Verification items for the finished model (mm, model axes). Face numbers are marked on the shaded views. A direction names the side the tool comes from. Round coordinates to 2 decimals unless told otherwise and drop trailing zeros. Write each loop counter-clockwise with the first axis right and the second up, starting at its lowest first coordinate (ties: lowest second). Pieces come first, ordered by that corner, then holes. Notation, with made-up numbers: (-29.75, -13) - (1.25, -13) arc R27 ccw to (1.25, 13) - close; hole circle Ø9 at (40.25, 28.25). An arc over 180 degrees is marked (long way). Write each question's results on one line, items separated by ' | '.
```python
from build123d import *

# Parameters (mm, degrees)
F1_DEPTH = 4
F3_DEPTH = 2
F4_R     = 1


with BuildPart() as f1:
    # F0 (on Top) → F1 (new body)
    with BuildSketch(Plane.XY):
        with BuildLine():
            ThreePointArc((-5, 0), (0, -5), (5, 0))
            ThreePointArc((5, 0), (0, 5), (-5, 0))
        make_face()
        Polygon((-4.041452, 0), (-2.020726, 3.5), (2.020726, 3.5), (4.041452, 0), (2.020726, -3.5), (-2.020726, -3.5), align=None, mode=Mode.SUBTRACT)
        with BuildLine():
            Line((5, -45), (5, 0))
            ThreePointArc((5, 0), (0, -5), (-5, 0))
            Line((-5, 0), (-5, -45))
            ThreePointArc((-5, -45), (0, -50), (5, -45))
        make_face()
    extrude(amount=F1_DEPTH)

    # F2 (on face) → F3 (cut)
    with BuildSketch(Plane.XY.offset(4)):
        with BuildLine():
            ThreePointArc((2.5, -9), (0, -6.5), (-2.5, -9))
            Line((-2.5, -9), (-2.5, -45))
            ThreePointArc((-2.5, -45), (0, -47.5), (2.5, -45))
            Line((2.5, -45), (2.5, -9))
        make_face()
    extrude(amount=-F3_DEPTH, mode=Mode.SUBTRACT)

    # F4
    f4_edges = [f1.edges().sort_by_distance(p)[0] for p in [
        (0, -6.5, 2),
        (-2.5, -27, 2),
        (0, -47.5, 2),
        (2.5, -27, 2),
    ]]
    fillet(f4_edges, radius=F4_R)


solid = f1.part
```
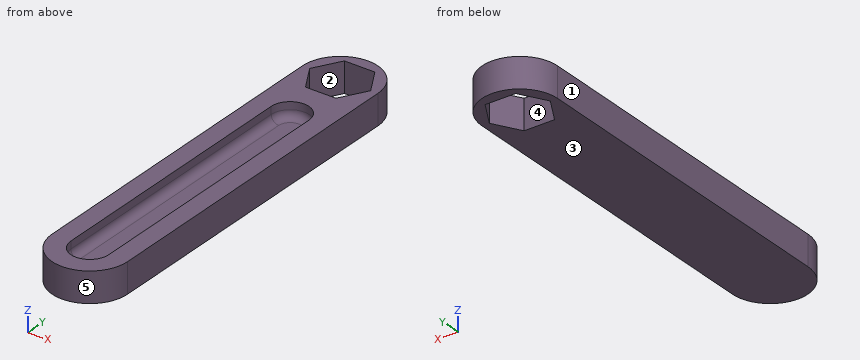
(1) Section check B-B (z = 1.3). Record the cut outline in (x, y), plus the area to 3 significant figures.
Answer:
outline: (-5, -45) arc R5 ccw to (5, -45) - (5, 0) arc R5 ccw to (-5, 0) - close; hole (-4.04, 0) - (-2.02, -3.5) - (2.02, -3.5) - (4.04, 0) - (2.02, 3.5) - (-2.02, 3.5) - close | area: 486 mm2
(2) Section check A-A (x = 0). Record the cut outline in (y, z).
Answer:
outline: (-50, 0) - (-3.5, 0) - (-3.5, 4) - (-6.5, 4) - (-6.5, 3) arc R1 cw to (-7.5, 2) - (-46.5, 2) arc R1 cw to (-47.5, 3) - (-47.5, 4) - (-50, 4) - close; (3.5, 0) - (5, 0) - (5, 4) - (3.5, 4) - close
(3) Mould release check, pull along X, two halves, no side actions. Record for the marked faces 1, 2 and 3: released by +X, released by -X, zero draft, split by the parting line, or undercut.
Answer:
face 1: released by -X | face 2: undercut | face 3: zero draft
(4) Set-up check for the marked faces 4 and 5: record each of +Z, -Z, +X, -X, +Y, -Y from which the full face is reachable in a straight line by a thin tool's end or side.
Answer:
face 4: +Z, -Z | face 5: +Z, -Z, -Y
(5) Section check D-D (y = -44.5). Record the cut outline in (x, z), plus the area to 3 significant figures.
Answer:
outline: (-5, 0) - (5, 0) - (5, 4) - (2.5, 4) - (2.5, 3) arc R1 cw to (1.5, 2) - (-1.5, 2) arc R1 cw to (-2.5, 3) - (-2.5, 4) - (-5, 4) - close | area: 30.4 mm2
(6) Go/stop test with flat-tipped pins: pin 1 Ø2.5 at (x, y) = (0, -22) entering from +Z; pin 2 Ø3 at (x, y) = (-0.5, -34) entering from +Z; pin 3 Ø1.5 at (x, z) = (-1.5, 1) entering from +Y. Record where each tip stops, or that it passes through.
Answer:
pin 1: z = 2 | pin 2: z = 2.13 | pin 3: y = 4.94
(7) Thickness scan on L1, parallel to X at y = 0, z = 3.7; L2, parallel to Y at x = -1, z = 3.35; L3, parallel to X at y = -11.5, z = 2.9. Record the ranges inside material, lowest first.
Answer:
L1: -5 to -4.04, 4.04 to 5 | L2: -49.9 to -47.29, -6.71 to -3.5, 3.5 to 4.9 | L3: -5 to -2.49, 2.49 to 5
(8) Section check C-C (y = -1). Record the cut outline in (x, z).
Answer:
outline: (-5, 0) - (-3.46, 0) - (-3.46, 4) - (-5, 4) - close; (3.46, 0) - (5, 0) - (5, 4) - (3.46, 4) - close
